```python
from build123d import *

# Parameters (mm, degrees)
SKETCH1_R           = 2.05
SKETCH1_R_2         = 6.55
BOSS_EXTRUDE1_DEPTH = 3.175
SKETCH2_W           = 10
SKETCH2_H           = 3.175
CUT_EXTRUDE1_DEPTH  = 3.175


with BuildPart() as part:
    # Sketch1 → Boss-Extrude1 (new body)
    with BuildSketch(Plane(origin=(0, 0, 0), x_dir=(1, 0, 0), z_dir=(0, 1, 0))):
        with BuildLine():
            ThreePointArc((-13.5, 51), (-26, 63.5), (-38.5, 51))
            Line((-38.5, 51), (-38.5, 38.5))
            Line((-38.5, 38.5), (-38.5, -38.5))
            Line((-38.5, -38.5), (38.5, -38.5))
            Line((38.5, -38.5), (51, -38.5))
            ThreePointArc((51, -38.5), (63.5, -26), (51, -13.5))
            Line((51, -13.5), (38.5, -13.5))
            Line((38.5, -13.5), (38.5, 38.5))
            Line((38.5, 38.5), (-13.5, 38.5))
            Line((-13.5, 38.5), (-13.5, 51))
        make_face()
        with Locations((41.475, -26)):
            Circle(SKETCH1_R, mode=Mode.SUBTRACT)
        with Locations((51, -35.525)):
            Circle(SKETCH1_R, mode=Mode.SUBTRACT)
        with Locations((51, -26)):
            Circle(SKETCH1_R_2, mode=Mode.SUBTRACT)
        with Locations((60.525, -26)):
            Circle(SKETCH1_R, mode=Mode.SUBTRACT)
        with Locations((-35.525, 51)):
            Circle(SKETCH1_R, mode=Mode.SUBTRACT)
        with Locations((-26, 41.475)):
            Circle(SKETCH1_R, mode=Mode.SUBTRACT)
        with Locations((-26, 51)):
            Circle(SKETCH1_R_2, mode=Mode.SUBTRACT)
        with Locations((-16.475, 51)):
            Circle(SKETCH1_R, mode=Mode.SUBTRACT)
        with Locations((-26, 60.525)):
            Circle(SKETCH1_R, mode=Mode.SUBTRACT)
        with Locations((51, -16.475)):
            Circle(SKETCH1_R, mode=Mode.SUBTRACT)
    extrude(amount=BOSS_EXTRUDE1_DEPTH)

    # Sketch2 → Cut-Extrude1 (cut)
    with BuildSketch(Plane(origin=(0, 3.175, 0), x_dir=(1, 0, 0), z_dir=(0, 1, 0))):
        with Locations((33.5, 36.9125)):
            Rectangle(SKETCH2_W, SKETCH2_H)
        with Locations((13.5, 36.9125)):
            Rectangle(SKETCH2_W, SKETCH2_H)
        with Locations((-6.5, 36.9125)):
            Rectangle(SKETCH2_W, SKETCH2_H)
        with Locations((-26.5, 36.9125)):
            Rectangle(SKETCH2_W, SKETCH2_H)
    extrude(amount=-CUT_EXTRUDE1_DEPTH, mode=Mode.SUBTRACT)


solid = part.part
```
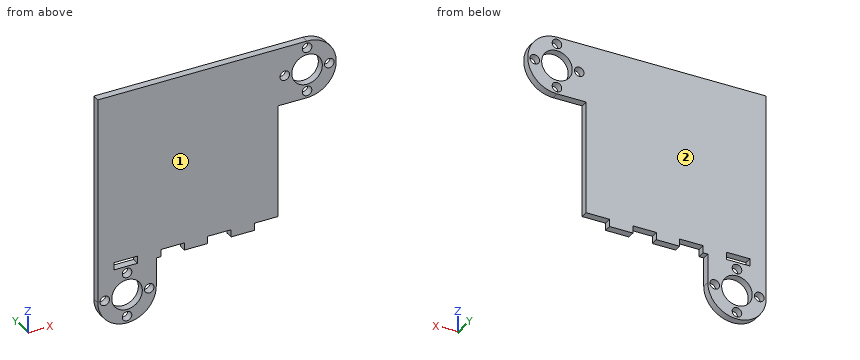
Input: part model. Units: mm. Frame: model coordinates. Face numbers are marked on the shaded views. Round coordinates to 2 decimals unless told otherwise and drop trailing zeros. Write each loop counter-clockwise with the first axis right and the second up, starting at its lowest first coordinate (ties: lowest second). Pieces come first, ordered by that corner, then holes. Notation, with made-up numbers: (56.5, 41.5) - (67.5, 41.5) arc R31 ccw to (67.5, 68.5) - close; hole circle Ø10 at (30, 88). An arc over 180 degrees is marked (long way). Write item = value, one per line.
(1) Material intervals for probe 1 along X at (y, z) = (2.1, 26) (3 decimals); probe 2 along Z at (x, y) = (51, 1.25) (3 decimals); probe 3 along Z at (x, y) = (-22.5, 1.65) (3 decimals), sorted ascending.
Geometry check:
probe_1 = -38.5 to 39.425, 43.525 to 44.45, 57.55 to 58.475, 62.575 to 63.5
probe_2 = 13.5 to 14.425, 18.525 to 19.45, 32.55 to 33.475, 37.575 to 38.5
probe_3 = -63 to -56.536, -45.464 to -38.5, -35.325 to 38.5
(2) Section query D-D on x = 6.5. Output: boundary loops of the cut face in (y, z) (3 decimals).
Geometry check:
outline = (0, -38.5) - (3.175, -38.5) - (3.175, 38.5) - (0, 38.5) - close
(3) Section query B-B on x = -26. Output: boundary loops of the cut face in (y, z) (3 decimals).
Geometry check:
outline = (0, -63.5) - (3.175, -63.5) - (3.175, -62.575) - (0, -62.575) - close; (0, -58.475) - (3.175, -58.475) - (3.175, -57.55) - (0, -57.55) - close; (0, -44.45) - (3.175, -44.45) - (3.175, -43.525) - (0, -43.525) - close; (0, -39.425) - (3.175, -39.425) - (3.175, -38.5) - (0, -38.5) - close; (0, -35.325) - (3.175, -35.325) - (3.175, 38.5) - (0, 38.5) - close
(4) Contact query for flat-ended pins moving along their axis: pin 1 Ø1 at (x, y) = (-4, 2.5) entering from -Z (3 decimals); pin 2 Ø1.6 at (x, y) = (26, 2.5) entering from -Z. Output: stop coordinate, or through.
Geometry check:
pin_1 = -35.325
pin_2 = -38.5
(5) Section query A-A on z = 26. Output: boundary loops of the cut face in (x, y) (3 decimals), then the cut area to 3 significant figures.
Geometry check:
outline = (-38.5, 0) - (39.425, 0) - (39.425, 3.175) - (-38.5, 3.175) - close; (43.525, 0) - (44.45, 0) - (44.45, 3.175) - (43.525, 3.175) - close; (57.55, 0) - (58.475, 0) - (58.475, 3.175) - (57.55, 3.175) - close; (62.575, 0) - (63.5, 0) - (63.5, 3.175) - (62.575, 3.175) - close
area = 256 mm^2
(6) Section query C-C on z = -36.5. Output: boundary loops of the cut face in (x, y) (3 decimals).
Geometry check:
outline = (-38.5, 0) - (-31.5, 0) - (-31.5, 3.175) - (-38.5, 3.175) - close; (-21.5, 0) - (-11.5, 0) - (-11.5, 3.175) - (-21.5, 3.175) - close; (-1.5, 0) - (8.5, 0) - (8.5, 3.175) - (-1.5, 3.175) - close; (18.5, 0) - (28.5, 0) - (28.5, 3.175) - (18.5, 3.175) - close
(7) Pull-direction query (Y, two-part tool) for the marked faces 1 and 2; classes: +Y half, -Y half, draft (parallel to the pull), parting line (faces both ways), or undercut.
Geometry check:
face_1 = -Y half
face_2 = +Y half
